For this review, take the finished solid that the model builds, in its own axes (mm). Face numbers are marked on the shaded views. A direction names the side the tool comes from. Coordinates: 2 decimals unless noted, no trailing zeros. Loops run counter-clockwise (first coordinate to the right, second up) from the corner with the lowest first, then second, coordinate; pieces in that order, holes last. Notation, with made-up numbers: (12, 66) -> (50, 66) arc R16 cw to (50, 78) -> close; hole circle Ø4 at (-22, -3). An arc over 180 degrees is marked (long way). Answer in a Markdown table with one row per item.
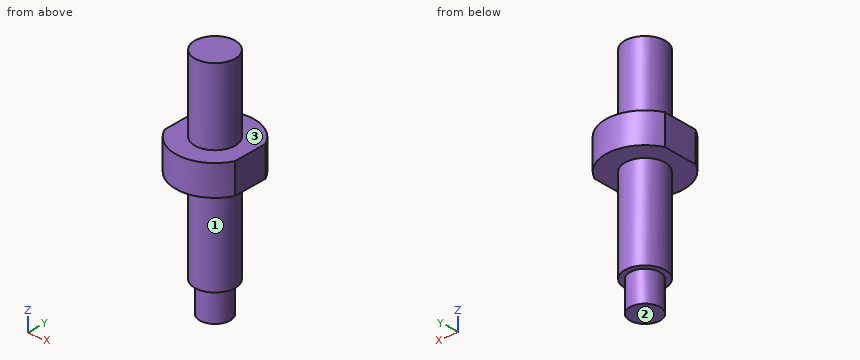
from build123d import *

# Parameters (mm, degrees)
SKETCH_3_W          = 8
SKETCH_3_H          = 16.823898374
CUT_EXTRUDE_1_DEPTH = 10
SKETCH_5_OUTSIDE_W  = 25.122
SKETCH_5_OUTSIDE_H  = 29.122
SKETCH_5_OUTSIDE_R  = 7.77784742
CUT_EXTRUDE_2_DEPTH = 10
SKETCH_6_R          = 3
EXTRUDE_1_DEPTH     = 6


with BuildPart() as part:
    # 草图2 → 旋转1 (revolve)
    with BuildSketch(Plane(origin=(0, 0, 0), x_dir=(0, 0, -1), z_dir=(1, 0, 0))):
        Polygon((0, 0), (0, 4), (15, 4), (15, 9), (21, 9), (21, 4), (39.5, 4), (39.5, 0), align=None)
    revolve(axis=Axis((0, 0, 0), (0, 0, -1)))

    # 草图3 → 切除-拉伸1 (cut)
    with BuildSketch(Plane.XY.offset(-15)):
        with Locations((-11, -0.026043186)):
            Rectangle(SKETCH_3_W, SKETCH_3_H)
        with Locations((11, -0.026043186)):
            Rectangle(SKETCH_3_W, SKETCH_3_H)
    extrude(amount=-CUT_EXTRUDE_1_DEPTH, mode=Mode.SUBTRACT)

    # 草图5 outside → 切除-拉伸2 (cut)
    with BuildSketch(Plane(origin=(0, 0, -21), x_dir=(-1, 0, 0), z_dir=(0, 0, -1))):
        Rectangle(SKETCH_5_OUTSIDE_W, SKETCH_5_OUTSIDE_H)
        Circle(SKETCH_5_OUTSIDE_R, mode=Mode.SUBTRACT)
    extrude(amount=-CUT_EXTRUDE_2_DEPTH, mode=Mode.SUBTRACT)

    # 草图6 → 凸台-拉伸1 (add)
    with BuildSketch(Plane(origin=(0, 0, -39.5), x_dir=(-1, 0, 0), z_dir=(0, 0, -1))):
        Circle(SKETCH_6_R)
    extrude(amount=EXTRUDE_1_DEPTH)


solid = part.part
Item 1: Take a section at B-B, the plane x = 0. State the section outline as (y, z) points, and give its area (3 significant figures).
Worked answers:
| item | result |
|---|---|
| outline | (-7.78, -21) -> (-4, -21) -> (-4, -39.5) -> (-3, -39.5) -> (-3, -45.5) -> (3, -45.5) -> (3, -39.5) -> (4, -39.5) -> (4, -21) -> (7.78, -21) -> (7.78, -15) -> (4, -15) -> (4, 0) -> (-4, 0) -> (-4, -15) -> (-7.78, -15) -> close |
| area | 397 mm² |
Item 2: Take a section at C-C, the plane z = -38.5. State the section outline as (x, y) points.
Worked answers:
| item | result |
|---|---|
| outline | circle Ø8 at (0, 0) |
Item 3: For L1, parallel to Y at x = 0.25, z = -22; L2, parallel to Z at x = -6, y = 2.25; L3, parallel to X at y = 0, z = -24.5, list the stretches that pass through material, from the lowest coordinate up.
Worked answers:
| item | result |
|---|---|
| L1 | -3.99 to 3.99 |
| L2 | -21 to -15 |
| L3 | -4 to 4 |
Item 4: For the marked faces 1, 2 and 3, list the 3-axis set-ups (+Z, -Z, +X, -X, +Y, -Y) from which the entire face can be reached by the end or side of a thin tool; tool diameter is ignored.
Worked answers:
| item | result |
|---|---|
| face 1 | -Z |
| face 2 | -Z, +X, -X, +Y, -Y |
| face 3 | +Z |
Item 5: Take a section at D-D, the plane y = 6.25. State the section outline as (x, z) points, and give its area (3 significant figures).
Worked answers:
| item | result |
|---|---|
| outline | (-4.63, -21) -> (4.63, -21) -> (4.63, -15) -> (-4.63, -15) -> close |
| area | 55.6 mm² |
Item 6: Insertion check: pin 1 (8 mm diameter, centred on y = 3, z = -40, fed in from +X); pin 2 (8 mm diameter, centred on x = -5.5, z = -4.5, fed in from +Y); pin 3 (2 mm diameter, centred on y = 4, z = -36, fed in from -X); pin 4 (1 mm diameter, centred on x = 5.5, z = -7, fed in from -Y) (3 decimals). Each pin has a flat end and moves straight along its axis. Give the tip position at first contact, or say it passes through.
Worked answers:
| item | result |
|---|---|
| pin 1 | x = 4 |
| pin 2 | y = 3.71 |
| pin 3 | x = -2.65 |
| pin 4 | through |
Item 7: Take a section at A-A, the plane y = 0. State the section outline as (x, z) points, and give its area (3 significant figures).
Worked answers:
| item | result |
|---|---|
| outline | (-7, -21) -> (-4, -21) -> (-4, -39.5) -> (-3, -39.5) -> (-3, -45.5) -> (3, -45.5) -> (3, -39.5) -> (4, -39.5) -> (4, -21) -> (7, -21) -> (7, -15) -> (4, -15) -> (4, 0) -> (-4, 0) -> (-4, -15) -> (-7, -15) -> close |
| area | 388 mm² |
